Autodesk Inventor part; units mm, degrees
ref_plane "YZ Plane" through (0, 0, 0) normal (1, 0, 0) x (0, 1, 0)
ref_plane "XZ Plane" through (0, 0, 0) normal (0, 1, 0) x (-1, 0, 0)
ref_plane "XY Plane" through (0, 0, 0) normal (0, 0, 1) x (1, 0, 0)
sketch "Esquisse1" plane through (0, 0, 0) normal (0, 0, 1) x (1, 0, 0)
  circle A0 centre (0, 0) radius 11.1
  dimension "d0" = 22.2
extrude "Extrusion1" add sketch "Esquisse1" along normal blind 13.4
sketch "Esquisse2" plane through (0, 0, 13.4) normal (0, 0, 1) x (1, 0, 0)
  circle A0 centre (0, 0) radius 11.1
  circle A1 centre (0, 0) radius 9.525
  dimension "d3" = 19.05
extrude "Extrusion2" cut sketch "Esquisse2" against normal blind 1.57
sketch "Esquisse4" plane through (0, 0, 13.4) normal (0, 0, 1) x (1, 0, 0)
  circle A0 centre (0, 0) radius 9.525
  circle A1 centre (0, 0) radius 1.585
  dimension "d7" = 3.17
extrude "Extrusion3" add sketch "Esquisse4" along normal blind 11.13 contours A1
properties part number "Vishay-157" material "Aluminium 6061"
Verification items for the finished model (mm, model axes). A direction names the side the tool comes from. Give positions to 0.01 mm unless a question says otherwise; leave off trailing zeros. Order: outer loops, then holes, each group sorted by start corner. A loop starts at its lowest first (then second) coordinate and runs counter-clockwise, first axis right, second up. Notation, with made-up numbers: M -22.75,24.5 L 9.25,24.5 A15 ccw 9.25,47.5 Z; hole C 15.5,34 d6. An arc over 180 degrees is marked long. Use one line per item in the form item = value. Start each with the question number.
Q1. Section check D-D (x = -7.25). Enter the section's corners in (y, z).
Q2. Access from +Z, -Z, +X, -X, +Y, -Y to the whole of each face (thin tool, end or side, straight path). Record for faces 1 (the flat face through (0, 0, 24.53)), 2 (the cylindrical face through (-1.26, 0.96, 18.89)).
Q3. Section check A-A (y = 0). Enter the section's corners in (x, z) (3 decimals).
Q4. Scan lines: line 1 along Z through (x, y) = (-3.5, -8.25); line 2 along Z through (x, y) = (-9, -3.5); line 3 along X through (y, z) = (-1, 3.5). Record each from-to range of solid material in increasing order. Write a range as [from, to].
Q5. Section check C-C (z = 9.5). Enter the section's corners in (x, y), then the cut area to 3 significant figures.
Q6. Go/stop test with flat-tipped pins: pin 1 Ø5 at (x, y) = (8, -1) entering from +Z; pin 2 Ø1.5 at (x, z) = (-2.5, 4) entering from -Y; pin 3 Ø2 at (x, z) = (-3, 3) entering from -Y. Record where each tip stops, or that it passes through.
Evaluation:
q1.outline = M -8.41,0 L 8.41,0 L 8.41,11.83 L 6.18,11.83 L 6.18,13.4 L -6.18,13.4 L -6.18,11.83 L -8.41,11.83 Z
q2.face_1 = +Z, +X, -X, +Y, -Y
q2.face_2 = +Z
q3.outline = M -11.1,0 L 11.1,0 L 11.1,11.83 L 9.525,11.83 L 9.525,13.4 L 1.585,13.4 L 1.585,24.53 L -1.585,24.53 L -1.585,13.4 L -9.525,13.4 L -9.525,11.83 L -11.1,11.83 Z
q4.line_1 = [0, 13.4]
q4.line_2 = [0, 11.83]
q4.line_3 = [-11.05, 11.05]
q5.outline = C 0,0 d22.2
q5.area = 387 mm2
q6.pin_1 = 13.4
q6.pin_2 = -10.96
q6.pin_3 = -10.92
